from build123d import *

# Parameters (mm, degrees)
SKETCH1_R           = 60
BOSS_EXTRUDE1_DEPTH = 2.4
SKETCH2_R           = 2.5
CUT_EXTRUDE1_DEPTH  = 85.988469806


with BuildPart() as part:
    # Sketch1 → Boss-Extrude1 (new, symmetric)
    with BuildSketch(Plane(origin=(0, 0, 0), x_dir=(1, 0, 0), z_dir=(0, 1, 0))):
        with Locations(Location((0, 0, 0), (0, 0, 270))):
            Circle(SKETCH1_R)
        Polygon((8.487048957, 0), (4.243524479, 7.35), (-4.243524479, 7.35), (-8.487048957, 0), (-4.243524479, -7.35), (4.243524479, -7.35), align=None, mode=Mode.SUBTRACT)
        Polygon((-14.780900235, -20), (-19.890450118, -11.15), (-30.109549882, -11.15), (-35.219099765, -20), (-30.109549882, -28.85), (-19.890450118, -28.85), align=None, mode=Mode.SUBTRACT)
        Polygon((35.219099765, -20), (30.109549882, -11.15), (19.890450118, -11.15), (14.780900235, -20), (19.890450118, -28.85), (30.109549882, -28.85), align=None, mode=Mode.SUBTRACT)
    extrude(amount=BOSS_EXTRUDE1_DEPTH, both=True)

    # Sketch2 → Cut-Extrude1 (cut, through all)
    with BuildSketch(Plane(origin=(0, 2.4, 0), x_dir=(1, 0, 0), z_dir=(0, 1, 0))):
        with Locations(Location((0, 35, 0), (0, 0, 270))):
            Circle(SKETCH2_R)
        with Locations(Location((17.65, 17.35, 0), (0, 0, 270))):
            Circle(SKETCH2_R)
        with Locations(Location((-17.65, 17.35, 0), (0, 0, 270))):
            Circle(SKETCH2_R)
    extrude(amount=-CUT_EXTRUDE1_DEPTH, mode=Mode.SUBTRACT)


solid = part.part
Input: part model. Units: mm. Frame: model coordinates. Coordinates: 2 decimals unless noted, no trailing zeros. Order: outer loops, then holes, each group sorted by start corner. A loop starts at its lowest first (then second) coordinate and runs counter-clockwise, first axis right, second up. Notation, with made-up numbers: M 58.25,-17 L 113.25,-17 A18 ccw 113.25,-8 Z; hole C -31.5,31 d1. An arc over 180 degrees is marked long. Answer as CSV lines item,"result".
1. Material intervals for line 1 (X direction, y = -1, z = -17.35); line 2 (Z direction, x = 0.5, y = 2); line 3 (Z direction, x = -16, y = 0.85), sorted ascending. Write a range as from..to.
Reported:
line 1,"-57.44..-20.15, -15.15..15.15, 20.15..57.44"
line 2,"-60..-37.45, -32.55..-7.35, 7.35..60"
line 3,"-57.83..-19.23, -15.47..17.89, 22.11..57.83"
2. Pull-direction query (Z, two-part tool) for faces 1 (the flat face through (-17.3, 0.03, 15.64)), 2 (the cylindrical face through (2.64, 0.03, -59.94)), 3 (the flat face through (-12, 2.4, -1)); classes: released by +Z, released by -Z, zero draft, split by the parting line, or undercut.
Reported:
face 1,"undercut"
face 2,"split by the parting line"
face 3,"zero draft"
3. Section A-A (x = 0). Return the cut outline in (y, z).
Reported:
outline,"M -2.4,-60 L 2.4,-60 L 2.4,-37.5 L -2.4,-37.5 Z; M -2.4,-32.5 L 2.4,-32.5 L 2.4,-7.35 L -2.4,-7.35 Z; M -2.4,7.35 L 2.4,7.35 L 2.4,60 L -2.4,60 Z"
4. Section C-C (x = 22.5). Return the cut outline in (y, z), then the cut area to 3 significant figures.
Reported:
outline,"M -2.4,-55.62 L 2.4,-55.62 L 2.4,11.15 L -2.4,11.15 Z; M -2.4,28.85 L 2.4,28.85 L 2.4,55.62 L -2.4,55.62 Z"
area,"449 mm2"
5. First-contact query: P1, Ø1.5, axis at y = -0.5, z = -41.5, coming from the +X side; P2, Ø2, axis at x = 44, y = 0.5, coming from the +Z side; P3, Ø1.5, axis at y = -0.5, z = 39, coming from the +X side. Flat tips, straight axial feed; report the tip coordinate or a pass-through.
Reported:
P1,"x = 44.04"
P2,"z = 41.84"
P3,"x = 46.23"
6. Section D-D (z = -35). Return the cut outline in (x, y).
Reported:
outline,"M -48.73,-2.4 L -2.5,-2.4 L -2.5,2.4 L -48.73,2.4 Z; M 2.5,-2.4 L 48.73,-2.4 L 48.73,2.4 L 2.5,2.4 Z"
7. Section B-B (y = -1.4). Return the cut outline in (x, z).
Reported:
outline,"C 0,0 d120; hole M -35.22,20 L -30.11,11.15 L -19.89,11.15 L -14.78,20 L -19.89,28.85 L -30.11,28.85 Z; hole C -17.65,-17.35 d5; hole M -8.49,0 L -4.24,-7.35 L 4.24,-7.35 L 8.49,0 L 4.24,7.35 L -4.24,7.35 Z; hole C 0,-35 d5; hole M 14.78,20 L 19.89,11.15 L 30.11,11.15 L 35.22,20 L 30.11,28.85 L 19.89,28.85 Z; hole C 17.65,-17.35 d5"
